```python
from build123d import *

# Parameters (mm, degrees)
BOSS_EXTRUDE1_DEPTH = 31
SKETCH2_W           = 5.5
SKETCH2_H           = 10.5
CUT_EXTRUDE1_DEPTH  = 7.5
SKETCH3_R           = 3
CUT_EXTRUDE2_DEPTH  = 7.5
CUT_EXTRUDE5_REACH  = 8.5
SKETCH6_W           = 8
SKETCH6_H           = 13
FILLET1_R           = 0.5
FILLET2_R           = 4
CUT_EXTRUDE7_REACH  = 27.5
SKETCH9_R           = 1.5
CUT_EXTRUDE8_DEPTH  = 17


with BuildPart() as part:
    # Sketch1 → Boss-Extrude1 (new body)
    with BuildSketch(Plane.XY):
        with BuildLine():
            Line((-3.75, 29), (-3.75, 22.5))
            Line((-3.75, 22.5), (-3.75, -22.5))
            Line((-3.75, -22.5), (2.75, -22.5))
            Line((2.75, -22.5), (2.75, 22.5))
            ThreePointArc((2.75, 22.5), (0.846194078, 27.096194078), (-3.75, 29))
        make_face()
    extrude(amount=BOSS_EXTRUDE1_DEPTH)

    # Sketch2 → Cut-Extrude1 (cut, through all)
    with BuildSketch(Plane.ZY.offset(3.75)):
        with Locations((28.25, 23.75)):
            Rectangle(SKETCH2_W, SKETCH2_H)
    extrude(amount=-CUT_EXTRUDE1_DEPTH, mode=Mode.SUBTRACT)

    # Sketch3 → Cut-Extrude2 (cut, through all)
    with BuildSketch(Plane.ZY.offset(3.75)):
        with Locations((21, 9)):
            Circle(SKETCH3_R)
        with Locations((21, -12.5)):
            Circle(SKETCH3_R)
    extrude(amount=-CUT_EXTRUDE2_DEPTH, mode=Mode.SUBTRACT)

    # Sketch6 → Cut-Extrude5 (cut, up to next)
    with BuildSketch(Plane.ZY.offset(3.75), mode=Mode.PRIVATE) as cut_extrude5_sk1:
        with Locations((4, 2)):
            Rectangle(SKETCH6_W, SKETCH6_H)
    cut_extrude5_tool1 = extrude(cut_extrude5_sk1.sketch, amount=-CUT_EXTRUDE5_REACH, mode=Mode.PRIVATE) & part.part
    add(cut_extrude5_tool1.solids().sort_by_distance((-3.75, 2, 4))[0], mode=Mode.SUBTRACT)

    # Fillet1
    fillet1_edges = [part.edges().sort_by_distance(p)[0] for p in [
        (-0.5, 8.5, 8),
        (-0.5, -4.5, 8),
    ]]
    fillet(fillet1_edges, radius=FILLET1_R)

    # Fillet2
    fillet2_edges = [part.edges().sort_by_distance(p)[0] for p in [
        (-0.5, -4.5, 0),
        (-0.5, 8.5, 0),
    ]]
    fillet(fillet2_edges, radius=FILLET2_R)

    # Sketch8 → Cut-Extrude7 (cut, up to next)
    with BuildSketch(Plane.XY.offset(25.5), mode=Mode.PRIVATE) as cut_extrude7_sk1:
        with BuildLine():
            Line((-3.75, 26.5), (-3.75, 18.5))
            ThreePointArc((-3.75, 18.5), (0.25, 22.5), (-3.75, 26.5))
        make_face()
    cut_extrude7_tool1 = extrude(cut_extrude7_sk1.sketch, amount=-CUT_EXTRUDE7_REACH, mode=Mode.PRIVATE) & part.part
    add(cut_extrude7_tool1.solids().sort_by_distance((-2.052347, 22.5, 25.5))[0], mode=Mode.SUBTRACT)

    # Sketch9 → Cut-Extrude8 (cut)
    with BuildSketch(Plane(origin=(0, 14.627294401, -2.055732165), x_dir=(-1, 0, 0), z_dir=(0, 0.990268069, -0.139173101))):
        with Locations((0.25, 29.426538121)):
            Circle(SKETCH9_R)
    extrude(amount=-CUT_EXTRUDE8_DEPTH, mode=Mode.SUBTRACT)


solid = part.part
```
Could you check a few things on this model? Use its own coordinates, in mm. A direction names the side the tool comes from. Round coordinates to 2 decimals unless told otherwise and drop trailing zeros. Loops run counter-clockwise (first coordinate to the right, second up) from the corner with the lowest first, then second, coordinate; pieces in that order, holes last. Notation, with made-up numbers: (75.5, 51) -> (126.5, 51) arc R21 cw to (126.5, 71) -> close; hole circle Ø2 at (84.5, 43.25). An arc over 180 degrees is marked (long way). Put each result on its own line as item: value.
Q1. I want a section at B-B on x = -3. Write out the boundary of the cut face in (y, z), and give its area (3 significant figures).
Checks:
outline: (-22.5, 0) -> (-8.5, 0) arc R4 ccw to (-4.5, 4) -> (-4.5, 7.5) arc R0.5 cw to (-4, 8) -> (8, 8) arc R0.5 cw to (8.5, 7.5) -> (8.5, 4) arc R4 ccw to (12.5, 0) -> (18.57, 0) -> (18.57, 25.5) -> (18.5, 25.5) -> (18.5, 31) -> (-22.5, 31) -> close; (26.43, 0) -> (28.96, 0) -> (28.96, 25.5) -> (26.43, 25.5) -> close; hole circle Ø6 at (-12.5, 21); hole circle Ø6 at (9, 21)
area: 1,170 mm2
Q2. Which directions (+Z, -Z, +X, -X, +Y, -Y) give clear straight access to the entire face, cutting with the end or side of a thin tool? Please do faces 1 (the flat face through (-1, -15, 0)), 2 (the flat face through (-0.23, 1.89, 29.47)), 3 (the cylindrical face through (0.896, 27.045, 12.572)), 4 (the cylindrical face through (-0.454, -5.641, 1.203)), 5 (the flat face through (1, 24, 25.5)).
Checks:
face 1: -Z, +X, -X, +Y, -Y
face 2: none
face 3: +Z, -Z, +X, +Y
face 4: -Z, +X, -X
face 5: +Z, +X, -X, +Y
Q3. I want a section at A-A on z = 21. Write out the boundary of the cut face in (x, y).
Checks:
outline: (-3.75, -22.5) -> (2.75, -22.5) -> (2.75, -15.5) -> (-3.75, -15.5) -> close; (-3.75, -9.5) -> (2.75, -9.5) -> (2.75, 6) -> (-3.75, 6) -> close; (-3.75, 12) -> (2.75, 12) -> (2.75, 22.5) arc R6.5 ccw to (-3.75, 29) -> (-3.75, 26.5) arc R4 cw to (-3.75, 18.5) -> close
Q4. Thinking about a two-plate mould opening in Z: for faces 6 (the cylindrical face through (-1, 10, 27)), 7 (the flat face through (-1, 2, 8)), 8 (the flat face through (-1, 8.5, 6)), which applies, pulls with the +Z half, pulls with the -Z half, needs draft (parallel to the pull), parting line crosses it, or undercut?
Checks:
face 6: undercut
face 7: pulls with the -Z half
face 8: needs draft
Q5. I want a section at D-D on z = 12.5. Write out the boundary of the cut face in (x, y), and give its area (3 significant figures).
Checks:
outline: (-3.75, -22.5) -> (2.75, -22.5) -> (2.75, 22.5) arc R6.5 ccw to (-3.75, 29) -> (-3.75, 26.5) arc R4 cw to (-3.75, 18.5) -> close
area: 301 mm2
Q6. Please list where these lines run through material, in increasing order: line 1 (Y direction, x = 0.5, z = 21); line 2 (Y direction, x = -1, z = 21); line 3 (Y direction, x = -3.25, z = 3). Write a range as from..to.
Checks:
line 1: -22.5..-15.5, -9.5..6, 12..27.42
line 2: -22.5..-15.5, -9.5..6, 12..19.6, 25.4..28.39
line 3: -22.5..-4.63, 8.63..18.53, 26.47..28.98
Q7. I want a section at C-C on y = -12.5. Write out the boundary of the cut face in (x, z), and give its area (4 significant figures).
Checks:
outline: (-3.75, 0) -> (2.75, 0) -> (2.75, 18) -> (-3.75, 18) -> close; (-3.75, 24) -> (2.75, 24) -> (2.75, 31) -> (-3.75, 31) -> close
area: 162.5 mm2
Q8. For pin 1 Ø2 at (x, y) = (-0.5, -1) entering from -Z; pin 2 Ø5.5 at (y, z) = (9, 21) entering from -X; pin 3 Ø1 at (x, z) = (-1.5, 20) entering from +Y; pin 4 Ø2 at (x, y) = (0.5, 22.5) entering from +Z, each with a flat end and sliding along its axis, tell me the tip position at first contact or that it passes through.
Checks:
pin 1: z = 8
pin 2: through
pin 3: y = 28.76
pin 4: z = 25.5
